from build123d import *

# Parameters (mm, degrees)
F0_R     = 10
F1_DEPTH = 10
F1_TAPER = 22.5
F4_T     = -0.4


with BuildPart() as f1:
    # F0 (on Top) → F1 (new body)
    with BuildSketch(Plane.XY):
        Circle(F0_R)
    extrude(amount=-F1_DEPTH, taper=F1_TAPER)

    # F2 (on Front) → F3 (revolve)
    with BuildSketch(Plane.XZ):
        with BuildLine():
            Line((0, 10), (0, 0))
            Line((0, 0), (10, 0))
            ThreePointArc((10, 0), (7.0710678119, 7.0710678119), (0, 10))
        make_face()
    revolve(axis=Axis((0, 0, -10), (0, 0, 1)))

    # F4
    f4_openings = [f1.faces().sort_by_distance(p)[0] for p in [
        (0, 0, -10),
    ]]
    offset(amount=F4_T, openings=f4_openings, kind=Kind.INTERSECTION)


solid = f1.part
Can you work these out from the model? Positions are in its coordinate system, mm. Give positions to 0.01 mm unless a question says otherwise; leave off trailing zeros. Order: outer loops, then holes, each group sorted by start corner. A loop starts at its lowest first (then second) coordinate and runs counter-clockwise, first axis right, second up. Notation, with made-up numbers: M 0,9 L 44,9 A5 ccw 44,17 Z; hole C 64.25,9.5 d9. An arc over 180 degrees is marked long. One line per question, with ' | ' between items.
Item 1: Please list where these lines run through material, in increasing order: L1, parallel to X at y = -7.25, z = 3; L2, parallel to X at y = -5.5, z = -3.5; L3, parallel to Y at x = -3.5, z = -7.
Answer block:
L1: x = -6.2 to -5.53, 5.53 to 6.2 | L2: x = -6.55 to -5.97, 5.97 to 6.55 | L3: y = -6.18 to -5.68, 5.68 to 6.18
Item 2: Suppose I cut it at B-B, the plane z = -7. Write out the boundary of the cut face in (x, y).
Answer block:
outline: C 0,0 d14.2; hole C 0,0 d13.34
Item 3: We'd pull the mould along Z, two halves only. Please class faces 1 (the face through (-1.42, -6.4, -7.27)), 2 (the face through (4, -4, -10)): released by +Z, released by -Z, zero draft, split by the parting line, or undercut.
Answer block:
face 1: undercut | face 2: released by -Z
Item 4: Suppose I cut it at C-C, the plane z = 2.5. Write out the boundary of the cut face in (x, y).
Answer block:
outline: C 0,0 d19.36; hole C 0,0 d18.54
Item 5: I'm going to push flat-ended pins straight in: pin 1 Ø2 at (x, z) = (-7.5, -6.5) entering from +Y; pin 2 Ø1.5 at (y, z) = (6, -7) entering from +X; pin 3 Ø1 at (x, z) = (1.5, 2) entering from +Y; pin 4 Ø1 at (x, y) = (7.5, 8) entering from +Z. Where does each tip first touch, or does it pass through?
Answer block:
pin 1: stops at y = 3.54 | pin 2: stops at x = 4.9 | pin 3: stops at y = 9.8 | pin 4: passes through
